Design review of the part built by this model. Coordinates are the model's own, in mm. A direction names the side the tool comes from. Round coordinates to 2 decimals unless told otherwise and drop trailing zeros. Return JSON: item names as keys, results as strings. Group by question number.
from build123d import *

# Parameters (mm, degrees)
SKETCH1_W           = 101.6
SKETCH1_H           = 152.4
BOSS_EXTRUDE1_DEPTH = 12.7
BOSS_EXTRUDE3_DEPTH = 12.7
FILLET1_R           = 2.54
FILLET2_R           = 5.08


with BuildPart() as part:
    # Sketch1 → Boss-Extrude1 (new body)
    with BuildSketch(Plane.XY):
        with Locations((50.8, 76.2)):
            Rectangle(SKETCH1_W, SKETCH1_H)
    extrude(amount=BOSS_EXTRUDE1_DEPTH)

    # Sketch2 → Boss-Extrude3 (add)
    with BuildSketch(Plane.XY):
        with BuildLine():
            add(Edge.make_bspline(
                [(0, 152.4), (39.790111277, 186.839065643), (12.30975625, 238.845497073), (0, 279.4)],
                knots=[0, 0, 0, 0, 1, 1, 1, 1], degree=3))
            add(Edge.make_bspline(
                [(0, 279.4), (51.286050257, 256.550041835), (87.836892382, 205.957944637), (101.6, 152.4)],
                knots=[0, 0, 0, 0, 1, 1, 1, 1], degree=3))
            Line((101.6, 152.4), (0, 152.4))
        make_face()
        with BuildLine():
            add(Edge.make_bspline(
                [(49.225838487, 233.315766274), (35.641228944, 236.267866949), (22.375615267, 231.937259722)],
                knots=[0, 0, 0, 1, 1, 1], degree=2))
            add(Edge.make_bspline(
                [(48.400350721, 207.535437601), (42.054170901, 227.566198031), (22.375615267, 231.937259722)],
                knots=[0, 0, 0, 1, 1, 1], degree=2))
            add(Edge.make_bspline(
                [(48.400350721, 207.535437601), (44.393568943, 220.734513873), (49.225838487, 233.315766274)],
                knots=[0, 0, 0, 1, 1, 1], degree=2))
        make_face(mode=Mode.SUBTRACT)
        with BuildLine():
            add(Edge.make_bspline(
                [(43.05348098, 206.08803494), (36.239789994, 218.91266054), (23.516066372, 224.861937296)],
                knots=[0, 0, 0, 1, 1, 1], degree=2))
            add(Edge.make_bspline(
                [(23.516066372, 224.861937296), (28.235295407, 215.21927262), (26.605728117, 204.582177714)],
                knots=[0, 0, 0, 1, 1, 1], degree=2))
            add(Edge.make_bspline(
                [(26.605728117, 204.582177714), (34.700432609, 206.792891754), (43.05348098, 206.08803494)],
                knots=[0, 0, 0, 1, 1, 1], degree=2))
        make_face(mode=Mode.SUBTRACT)
        with BuildLine():
            add(Edge.make_bspline(
                [(82.396089655, 183.81371778), (70.6713649, 174.663598784), (70.32777317, 160.02)],
                knots=[0, 0, 0, 1, 1, 1], degree=2))
            Line((70.32777317, 160.02), (87.546521436, 160.02))
            add(Edge.make_bspline(
                [(82.396089655, 183.81371778), (89.339550367, 172.773814043), (87.546521436, 160.02)],
                knots=[0, 0, 0, 1, 1, 1], degree=2))
        make_face(mode=Mode.SUBTRACT)
        with BuildLine():
            add(Edge.make_bspline(
                [(26.980466376, 183.81374211), (28.958775605, 170.837543608), (21.602944743, 160.02)],
                knots=[0, 0, 0, 1, 1, 1], degree=2))
            Line((21.602944743, 160.02), (40.676641776, 160.02))
            add(Edge.make_bspline(
                [(26.980466376, 183.81374211), (36.13847285, 173.175056715), (40.676641776, 160.02)],
                knots=[0, 0, 0, 1, 1, 1], degree=2))
        make_face(mode=Mode.SUBTRACT)
        with BuildLine():
            add(Edge.make_bspline(
                [(54.97708308, 160.02), (46.08347584, 181.54755316), (28.342136903, 196.529802482)],
                knots=[0, 0, 0, 1, 1, 1], degree=2))
            add(Edge.make_bspline(
                [(28.342136903, 196.529802482), (53.017815002, 201.732288521), (77.187204495, 194.363538628)],
                knots=[0, 0, 0, 1, 1, 1], degree=2))
            add(Edge.make_bspline(
                [(54.97708308, 160.02), (59.374728895, 181.400643158), (77.187204495, 194.363538628)],
                knots=[0, 0, 0, 1, 1, 1], degree=2))
        make_face(mode=Mode.SUBTRACT)
        with BuildLine():
            add(Edge.make_bspline(
                [(70.328259561, 206.277457578), (62.361576962, 208.669014941), (54.287141362, 207.109917469)],
                knots=[0, 0, 0, 1, 1, 1], degree=2))
            add(Edge.make_bspline(
                [(54.287141362, 207.109917469), (53.482096811, 217.391663167), (54.97708308, 227.557269012)],
                knots=[0, 0, 0, 1, 1, 1], degree=2))
            add(Edge.make_bspline(
                [(54.97708308, 227.557269012), (66.645859754, 219.852180834), (70.328259561, 206.277457578)],
                knots=[0, 0, 0, 1, 1, 1], degree=2))
        make_face(mode=Mode.SUBTRACT)
        with BuildLine():
            add(Edge.make_bspline(
                [(21.602944743, 238.323137826), (19.95197567, 252.974545225), (11.094737768, 264.601494061)],
                knots=[0, 0, 0, 1, 1, 1], degree=2))
            add(Edge.make_bspline(
                [(11.094737768, 264.601494061), (28.053835186, 259.295838115), (38.412267282, 244.949944056)],
                knots=[0, 0, 0, 1, 1, 1], degree=2))
            add(Edge.make_bspline(
                [(21.602944743, 238.323137826), (31.864782779, 237.284469605), (38.412267282, 244.949944056)],
                knots=[0, 0, 0, 1, 1, 1], degree=2))
        make_face(mode=Mode.SUBTRACT)
    extrude(amount=BOSS_EXTRUDE3_DEPTH)

    # Fillet1
    fillet1_edges = [part.edges().sort_by_distance(p)[0] for p in [
        (101.6, 152.4, 6.35),
        (0, 152.4, 6.35),
    ]]
    fillet(fillet1_edges, radius=FILLET1_R)

    # Fillet2
    fillet2_edges = [part.edges().sort_by_distance(p)[0] for p in [
        (0, 0, 6.35),
        (101.6, 0, 6.35),
    ]]
    fillet(fillet2_edges, radius=FILLET2_R)


solid = part.part
Q1. Tool access review of faces 1 (the flat face through (31, 160.02, 6)), 2 (the flat face through (52, 111, 0)): name each direction out of +Z, -Z, +X, -X, +Y, -Y from which nothing blocks a thin tool from reaching the whole face with its end or side.
Q2. For line 1 (Y direction, x = 67, z = 7.5); line 2 (Y direction, x = 58.5, z = 12) (3 decimals); line 3 (X direction, y = 167.5, z = 5.5), list the stretches that pass through material, from the lowest coordinate up.
Q3. Insertion check: pin 1 Ø4 at (x, y) = (62.5, 216) entering from +Z; pin 2 Ø1.5 at (x, z) = (64, 4.5) entering from +Y; pin 3 Ø6.5 at (x, z) = (27, 9) entering from +Y; pin 4 Ø4 at (x, y) = (27.5, 204) entering from -Z. Each pin has a flat end and moves straight along its axis. Give the tip position at first contact, or say it passes through.
Q4. Add section A-A, the plane z = 2.75. Give the number of separate pieces and of enclosed holes in the cut face, plus the area to 3 significant figures.
Evaluation:
{
 "1": {"face 1": "+Z, -Z", "face 2": "-Z, +X, -X, +Y, -Y"},
 "2": {"line 1": "0 to 185.02, 196.91 to 207.1, 214.65 to 224.63", "line 2": "0 to 171.353, 198.174 to 207.655, 224.947 to 235.182", "line 3": "12.8 to 25.48, 37.63 to 51.52, 57.01 to 71.34, 87.84 to 97.09"},
 "3": {"pin 1": "through", "pin 2": "y = 229.47", "pin 3": "y = 266.2", "pin 4": "z = 0"},
 "4": {"separate pieces": "1", "enclosed holes": "7", "area": "20,000 mm²"}
}
